Check sheet for the modelled part. Datum: model origin and axes. Units: mm. Round coordinates to 2 decimals unless told otherwise and drop trailing zeros. Loops run counter-clockwise (first coordinate to the right, second up) from the corner with the lowest first, then second, coordinate; pieces in that order, holes last. Notation, with made-up numbers: (39, 18) -> (89, 18) arc R14 ccw to (89, 37) -> close; hole circle Ø2 at (-38.5, -30.5). An arc over 180 degrees is marked (long way). One line per question, with ' | ' between items.
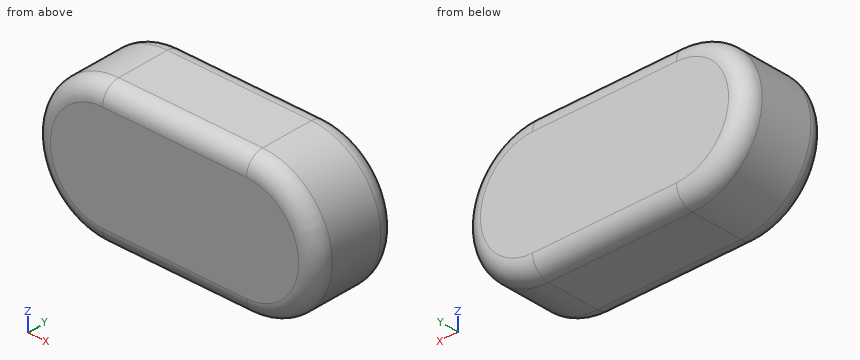
```python
from build123d import *

# Parameters (mm, degrees)
F1_DEPTH = 12.5
F2_R     = 5


with BuildPart() as f1:
    # F0 (on Front) → F1 (new body, symmetric)
    with BuildSketch(Plane.XZ):
        with BuildLine():
            ThreePointArc((-18.81171, 20), (-38.81171, 0), (-18.81171, -20))
            Line((-18.81171, -20), (22.574065, -20))
            ThreePointArc((22.574065, -20), (42.574065, 0), (22.574065, 20))
            Line((22.574065, 20), (-18.81171, 20))
        make_face()
    extrude(amount=F1_DEPTH, both=True)

    # F2
    f2_edges = [f1.edges().sort_by_distance(p)[0] for p in [
        (42.574065, -12.5, 0),
        (42.574065, 12.5, 0),
    ]]
    fillet(f2_edges, radius=F2_R)


solid = f1.part
```
(1) Sectioned sample at B-B, the plane y = -1. Record the cut outline in (x, z), and give its area (3 significant figures).
Answer:
outline: (-18.81, -20) -> (22.57, -20) arc R20 ccw to (22.57, 20) -> (-18.81, 20) arc R20 ccw to start | area: 2,910 mm2
(2) Sectioned sample at A-A, the plane x = 0. Record the cut outline in (y, z), and give its area (3 significant figures).
Answer:
outline: (-12.5, -15) arc R5 ccw to (-7.5, -20) -> (7.5, -20) arc R5 ccw to (12.5, -15) -> (12.5, 15) arc R5 ccw to (7.5, 20) -> (-7.5, 20) arc R5 ccw to (-12.5, 15) -> close | area: 979 mm2
(3) Scan lines: probe 1 along X at (y, z) = (-1, 1); probe 2 along Y at (x, z) = (1.5, 17); probe 3 along Y at (x, z) = (33.5, 11). Record each from-to range of solid material in increasing order.
Answer:
probe 1: x = -38.79 to 42.55 | probe 2: y = -12.08 to 12.08 | probe 3: y = -12.47 to 12.47
(4) Sectioned sample at C-C, the plane y = -10.75. Record the cut outline in (x, z), and give its area (3 significant figures).
Answer:
outline: (-18.81, -18.8) -> (22.57, -18.8) arc R18.8 ccw to (22.57, 18.8) -> (-18.81, 18.8) arc R18.8 ccw to start | area: 2,670 mm2
(5) Go/stop test with flat-tipped pins: pin 1 (6 mm diameter, centred on y = -3.5, z = 7.5, fed in from -X); pin 2 (3 mm diameter, centred on y = -2, z = 16, fed in from +X); pin 3 (12 mm diameter, centred on y = 5, z = 9, fed in from -X). Record where each tip stops, or that it passes through.
Answer:
pin 1: stops at x = -38.3 | pin 2: stops at x = 36.35 | pin 3: stops at x = -38.59
